The listing builds one solid part. Answer for the finished solid, in the listing's coordinates (mm). Round coordinates to 2 decimals unless told otherwise and drop trailing zeros. Write item = value, one per line.
from build123d import *

# Parameters (mm, degrees)
F0_W     = 400
F0_H     = 350
F1_DEPTH = 19
F3_DEPTH = 25
F2_R     = 32.5444100718
F4_DEPTH = 25


with BuildPart() as f1:
    # F0 (on Top) → F1 (new body)
    with BuildSketch(Plane.XY):
        Rectangle(F0_W, F0_H)
    extrude(amount=F1_DEPTH)

    # F2 (on face) → F3 (cut)
    with BuildSketch(Plane.XY.offset(19)):
        with BuildLine():
            Line((200, 175), (1.2303346045, 175))
            add(Edge.make_bspline(
                [(200, 1.2037944383), (199.5351083689, 87.0242167051), (99.8085920468, 174.6364886784), (1.2303346045, 175)],
                knots=[0.7494961922, 0.7494961922, 0.7494961922, 0.7494961922, 0.9989620997, 0.9989620997, 0.9989620997, 0.9989620997], degree=3))
            Line((200, 1.2037944383), (200, 175))
        make_face()
        with BuildLine():
            add(Edge.make_bspline(
                [(0, 175), (-98.8187558399, 174.6350450151), (-292.6120906446, -1.5966892013), (-0.9342373868, -252.8984666735), (199.5335407467, -85.9557258275), (200, 0)],
                knots=[0, 0, 0, 0, 0.2501031726, 0.4984159764, 0.7483296585, 0.7483296585, 0.7483296585, 0.7483296585], degree=3))
            Line((0, 175), (-200, 175))
            Line((-200, 175), (-200, -175))
            Line((-200, -175), (200, -175))
            Line((200, -175), (200, 0))
        make_face()
    extrude(amount=-F3_DEPTH, mode=Mode.SUBTRACT)

    # F2 (on face) → F4 (cut)
    with BuildSketch(Plane.XY.offset(19)):
        with Locations((-75.0856101513, 112.3721450567)):
            Circle(F2_R)
    extrude(amount=-F4_DEPTH, mode=Mode.SUBTRACT)


solid = f1.part
Q1. Determine the mould class of faces 1 (the face through (5, 12, 19)), 2 (the face through (-45.02, 99.91, 9.63)) for opening direction X: released by +X, released by -X, zero draft, split by the parting line, or undercut.
Model answer:
face_1 = zero draft
face_2 = undercut
Q2. Flat-ended cylindrical pins translate along their axes: P1, Ø8, axis at y = 89.5, z = 4, coming from the -X side; P2, Ø8, axis at x = -79.5, z = 4, coming from the -Y side; P3, Ø8, axis at y = 60, z = 16.5, coming from the +X side. Find the tip coordinate at first contact, or state that the pin passes through.
Model answer:
P1 = -165.72
P2 = -153.31
P3 = 186.9
Q3. Find the intervals of material crossed by line 1 (Y direction, x = -1, z = 11.25); line 2 (Y direction, x = -47.5, z = 17.5); line 3 (Y direction, x = -69, z = 16.5), in increasing order. Write a range as from..to.
Model answer:
line_1 = -169.33..174.99
line_2 = -162.9..95.1, 129.64..168.27
line_3 = -155.93..80.4, 144.34..160.99
